Design review of the part built by this model. Coordinates are the model's own, in mm. Face numbers are marked on the shaded views. Give positions to 0.01 mm unless a question says otherwise; leave off trailing zeros. Write each loop counter-clockwise with the first axis right and the second up, starting at its lowest first coordinate (ties: lowest second). Pieces come first, ordered by that corner, then holes.
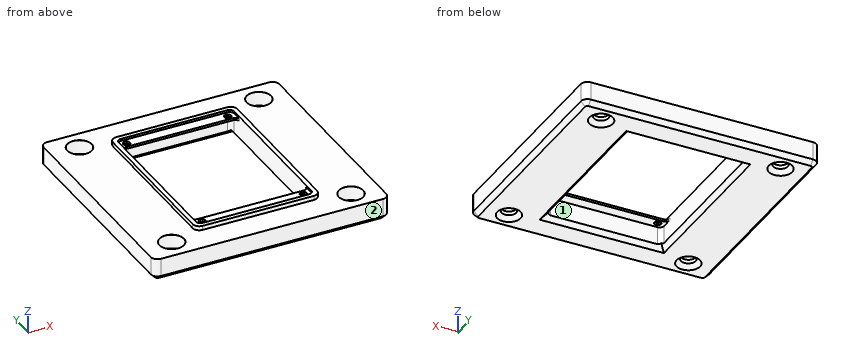
```python
from build123d import *

# Parameters (mm, degrees)
BOSS_EXTRUDE3_DEPTH                          = 10
BOSS_EXTRUDE3_DEPTH_BACK                     = 0.1
SKETCH1_W                                    = 100
SKETCH1_H                                    = 106
SKETCH1_W_2                                  = 76
SKETCH1_H_2                                  = 56
CBORE_FOR_M6_HEX_SOCKET_HEAD_CAP_SCR_2_COUNT = 2
CBORE_FOR_M6_HEX_SOCKET_HEAD_CAP_SCR_2_PITCH = 81
CBORE_FOR_M6_HEX_SOCKET_HEAD_CAP_SCR_3_COUNT = 2
CBORE_FOR_M6_HEX_SOCKET_HEAD_CAP_SCR_3_PITCH = 114.385386776
CBORE_FOR_M6_HEX_SOCKET_HEAD_CAP_SCR_4_COUNT = 2
CBORE_FOR_M6_HEX_SOCKET_HEAD_CAP_SCR_4_PITCH = 80.765194904
SKETCH7_W                                    = 56
SKETCH7_H                                    = 76
BOSS_EXTRUDE4_DEPTH                          = 12
SKETCH8_W                                    = 52
SKETCH8_H                                    = 72
BOSS_EXTRUDE5_DEPTH                          = 1
SKETCH9_W                                    = 52
SKETCH9_H                                    = 72
CUT_EXTRUDE1_DEPTH                           = 1
SKETCH10_W                                   = 52
SKETCH10_H                                   = 62.005454301
CUT_EXTRUDE2_DEPTH                           = 11
SKETCH11_W                                   = 52
SKETCH11_H                                   = 4.999168043
SKETCH11_H_2                                 = 4.995377656
CUT_EXTRUDE3_DEPTH                           = 10
SKETCH12_R                                   = 1.5
CUT_EXTRUDE4_DEPTH                           = 2
SKETCH12_3_R                                 = 1.5
CUT_EXTRUDE5_DEPTH                           = 2
SKETCH14_R                                   = 1.5
CUT_EXTRUDE6_DEPTH                           = 2
SKETCH15_R                                   = 1.5
CUT_EXTRUDE7_DEPTH                           = 2
FILLET2_R                                    = 3
CHAMFER1_SIZE                                = 2
FILLET3_R                                    = 2
FILLET4_R                                    = 2


with BuildPart() as part:
    # Sketch1 → Boss-Extrude3 (new, two sides: drawn at the far end of the back side and taken through both)
    # profile 1 of 4: a face of its own
    with BuildSketch(Plane(origin=(0, 0, 0), x_dir=(0, 1, 0), z_dir=(0, 0, 1)).offset(-BOSS_EXTRUDE3_DEPTH_BACK)):
        with Locations((-4.589836902, -8.848323211)):
            Rectangle(SKETCH1_W, SKETCH1_H)
        with Locations((-4.589836902, -8.848323211)):
            Rectangle(SKETCH1_W_2, SKETCH1_H_2, mode=Mode.SUBTRACT)
    # profile 2 of 4: a face of its own
    with BuildSketch(Plane(origin=(0, 0, 0), x_dir=(0, 1, 0), z_dir=(0, 0, 1)).offset(-BOSS_EXTRUDE3_DEPTH_BACK)):
        Polygon((39.410163098, 31.651676789), (39.410163098, -49.348323211), (45.410163098, -61.848323211), (45.410163098, 44.151676789), align=None)
    # profile 3 of 4: a face of its own
    with BuildSketch(Plane(origin=(0, 0, 0), x_dir=(0, 1, 0), z_dir=(0, 0, 1)).offset(-BOSS_EXTRUDE3_DEPTH_BACK)):
        Polygon((33.410163098, 19.151676789), (33.410163098, -36.848323211), (39.410163098, -49.348323211), (39.410163098, 31.651676789), align=None)
    # profile 4 of 4: a face of its own
    with BuildSketch(Plane(origin=(0, 0, 0), x_dir=(0, 1, 0), z_dir=(0, 0, 1)).offset(-BOSS_EXTRUDE3_DEPTH_BACK)):
        Polygon((45.410163098, -61.848323211), (39.410163098, -49.348323211), (39.410163098, -61.848323211), align=None)
    extrude(amount=BOSS_EXTRUDE3_DEPTH + BOSS_EXTRUDE3_DEPTH_BACK)

    # Sketch6 → CBORE for M6 Hex Socket Head Cap Screw2 (revolve, cut)
    with BuildSketch(Plane(origin=(49.348323211, -45.089836902, 10), x_dir=(0, -1, 0), z_dir=(1, 0, 0))):
        Polygon((0, 0), (0, 10.1), (3.3, 10.1), (3.3, 6.4), (5.5, 6.4), (5.5, 0.025), (5.525, 0), align=None)
    cbore_for_m6_hex_socket_head_cap_screw2 = revolve(axis=Axis((49.348323211, -45.089836902, 16.35), (0, 0, -1)), mode=Mode.SUBTRACT)

    # CBORE for M6 Hex Socket Head Cap Scr 2: CBORE for M6 Hex Socket Head Cap Screw2 ×2
    with Locations(*[(0, i * CBORE_FOR_M6_HEX_SOCKET_HEAD_CAP_SCR_2_PITCH, 0) for i in range(1, CBORE_FOR_M6_HEX_SOCKET_HEAD_CAP_SCR_2_COUNT)]):
        add(cbore_for_m6_hex_socket_head_cap_screw2, mode=Mode.SUBTRACT)

    # CBORE for M6 Hex Socket Head Cap Scr 3: CBORE for M6 Hex Socket Head Cap Screw2 ×2
    with Locations(*[Vector(-0.7060796591298035, 0.7081324134391396, 0) * (i * CBORE_FOR_M6_HEX_SOCKET_HEAD_CAP_SCR_3_PITCH) for i in range(1, CBORE_FOR_M6_HEX_SOCKET_HEAD_CAP_SCR_3_COUNT)]):
        add(cbore_for_m6_hex_socket_head_cap_screw2, mode=Mode.SUBTRACT)

    # CBORE for M6 Hex Socket Head Cap Scr 4: CBORE for M6 Hex Socket Head Cap Screw2 ×2
    with Locations(*[(-i * CBORE_FOR_M6_HEX_SOCKET_HEAD_CAP_SCR_4_PITCH, 0, 0) for i in range(1, CBORE_FOR_M6_HEX_SOCKET_HEAD_CAP_SCR_4_COUNT)]):
        add(cbore_for_m6_hex_socket_head_cap_screw2, mode=Mode.SUBTRACT)

    # Sketch7 → Boss-Extrude4 (add)
    with BuildSketch(Plane(origin=(0, 0, -0.1), x_dir=(1, 0, 0), z_dir=(0, 0, -1))):
        with Locations((8.848323211, 4.589836902)):
            Rectangle(SKETCH7_W, SKETCH7_H)
    extrude(amount=-BOSS_EXTRUDE4_DEPTH)

    # Sketch8 → Boss-Extrude5 (add)
    with BuildSketch(Plane.XY.offset(11.9)):
        with Locations((8.848323211, -4.589836902)):
            Rectangle(SKETCH8_W, SKETCH8_H)
    extrude(amount=-BOSS_EXTRUDE5_DEPTH)

    # Sketch9 → Cut-Extrude1 (cut)
    with BuildSketch(Plane.XY.offset(11.9)):
        with Locations((8.848323211, -4.589836902)):
            Rectangle(SKETCH9_W, SKETCH9_H)
    extrude(amount=-CUT_EXTRUDE1_DEPTH, mode=Mode.SUBTRACT)

    # Sketch10 → Cut-Extrude2 (cut)
    with BuildSketch(Plane.XY.offset(10.9)):
        with Locations((8.848323211, -4.587941709)):
            Rectangle(SKETCH10_W, SKETCH10_H)
    extrude(amount=-CUT_EXTRUDE2_DEPTH, mode=Mode.SUBTRACT)

    # Sketch11 → Cut-Extrude3 (cut)
    with BuildSketch(Plane(origin=(0, 0, -0.1), x_dir=(1, 0, 0), z_dir=(0, 0, -1))):
        with Locations((8.848323211, 38.090252881)):
            Rectangle(SKETCH11_W, SKETCH11_H)
        with Locations((8.848323211, -28.91247427)):
            Rectangle(SKETCH11_W, SKETCH11_H_2)
    extrude(amount=-CUT_EXTRUDE3_DEPTH, mode=Mode.SUBTRACT)

    # Sketch12 → Cut-Extrude4 (cut)
    with BuildSketch(Plane.XY.offset(10.9)):
        with Locations((-13.901676789, 28.660163098)):
            Circle(SKETCH12_R)
    extrude(amount=-CUT_EXTRUDE4_DEPTH, mode=Mode.SUBTRACT)

    # Sketch12_3 → Cut-Extrude5 (cut)
    with BuildSketch(Plane.XY.offset(10.9)):
        with Locations((31.598323211, 28.660163098)):
            Circle(SKETCH12_3_R)
    extrude(amount=-CUT_EXTRUDE5_DEPTH, mode=Mode.SUBTRACT)

    # Sketch14 → Cut-Extrude6 (cut)
    with BuildSketch(Plane.XY.offset(10.9)):
        with Locations((-13.901676789, -37.839836902)):
            Circle(SKETCH14_R)
    extrude(amount=-CUT_EXTRUDE6_DEPTH, mode=Mode.SUBTRACT)

    # Sketch15 → Cut-Extrude7 (cut)
    with BuildSketch(Plane.XY.offset(10.9)):
        with Locations((31.598323211, -37.839836902)):
            Circle(SKETCH15_R)
    extrude(amount=-CUT_EXTRUDE7_DEPTH, mode=Mode.SUBTRACT)

    # Fillet2
    fillet2_edges = [part.edges().sort_by_distance(p)[0] for p in [
        (61.848323211, -54.589836902, 4.95),
        (-44.151676789, -54.589836902, 4.95),
        (-44.151676789, 45.410163098, 4.95),
        (61.848323211, 45.410163098, 4.95),
        (-19.151676789, 33.410163098, 10.95),
        (-19.151676789, -42.589836902, 10.95),
        (36.848323211, -42.589836902, 10.95),
        (36.848323211, 33.410163098, 10.95),
    ]]
    fillet(fillet2_edges, radius=FILLET2_R)

    # Chamfer1
    chamfer1_edges = [part.edges().sort_by_distance(p)[0] for p in [
        (-17.151676789, -4.589836902, -0.1),
        (34.848323211, -4.589836902, -0.1),
        (8.848323211, -40.589836902, -0.1),
        (8.848323211, 31.410163098, -0.1),
        (8.848323211, 45.410163098, -0.1),
        (-44.151676789, -4.589836902, -0.1),
        (61.848323211, -4.589836902, -0.1),
        (8.848323211, -54.589836902, -0.1),
        (-43.272997132, -53.711157246, -0.1),
        (60.969643555, -53.711157246, -0.1),
        (60.969643555, 44.531483441, -0.1),
        (-43.272997132, 44.531483441, -0.1),
        (49.348323211, -41.789836902, -0.1),
        (-31.416871693, -41.789836902, -0.1),
        (-31.416871693, 39.210163098, -0.1),
        (49.348323211, 39.210163098, -0.1),
    ]]
    chamfer(chamfer1_edges, length=CHAMFER1_SIZE)

    # Fillet3
    fillet3_edges = [part.edges().sort_by_distance(p)[0] for p in [
        (34.848323211, -35.590668859, 10.4),
    ]]
    fillet(fillet3_edges, radius=FILLET3_R)

    # Fillet4
    fillet4_edges = [part.edges().sort_by_distance(p)[0] for p in [
        (-17.151676789, -40.589836902, 11.4),
        (-17.151676789, 31.410163098, 11.4),
        (34.848323211, 31.410163098, 11.4),
        (34.848323211, -40.589836902, 11.4),
        (-17.151676789, 26.414785442, 10.4),
        (34.848323211, 26.414785442, 10.4),
        (-17.151676789, -35.590668859, 10.4),
        (-17.151676789, -40.589836902, 5.9),
        (34.848323211, -40.589836902, 5.9),
        (34.848323211, 31.410163098, 5.9),
        (-17.151676789, 31.410163098, 5.9),
    ]]
    fillet(fillet4_edges, radius=FILLET4_R)


solid = part.part
```
(1) Clearance check with flat-ended pins moving along their axes: P1, Ø12, axis at x = 47.5, y = -47.5, coming from the +Z side; P2, Ø5, axis at x = 31.6, y = -37.84, coming from the -Z side; P3, Ø1, axis at y = 2.5, z = 11.5, coming from the -X side. State where each tip first meets the part, or that it passes through.
Resolved:
P1: stops at z = 10
P2: stops at z = 9.9
P3: stops at x = -19.15
(2) Mouldability with a two-part tool opening along X and no side actions: class the marked faces 1 and 2 as pulls with the +X half, pulls with the -X half, needs draft (parallel to the pull), parting line crosses it, or undercut.
Resolved:
face 1: undercut
face 2: needs draft
(3) Consider section A-A, the plane y = 19. Give the boundary of the cut face in (x, z).
Resolved:
outline: (-44.15, 1.9) - (-42.15, -0.1) - (-19.15, -0.1) - (-17.15, 1.9) - (-17.15, 11.9) - (-19.15, 11.9) - (-19.15, 10) - (-44.15, 10) - close; (34.85, 1.9) - (36.85, -0.1) - (59.85, -0.1) - (61.85, 1.9) - (61.85, 10) - (36.85, 10) - (36.85, 11.9) - (34.85, 11.9) - close
(4) Consider section C-C, the plane x = 31.5. Give the number of separate pieces and of enclosed holes in the cut face, then the cut area to 3 significant figures.
Resolved:
separate pieces: 4
enclosed holes: 0
area: 286 mm2
(5) Consider section D-D, the plane z = 5.75. Give the boundary of the cut face in (x, y).
Resolved:
outline: (-44.15, -51.59) arc R3 ccw to (-41.15, -54.59) - (58.85, -54.59) arc R3 ccw to (61.85, -51.59) - (61.85, 42.41) arc R3 ccw to (58.85, 45.41) - (-41.15, 45.41) arc R3 ccw to (-44.15, 42.41) - close; hole circle Ø11 at (-31.42, -45.09); hole circle Ø11 at (-31.42, 35.91); hole (-17.15, -38.59) arc R2 ccw to (-15.15, -40.59) - (32.85, -40.59) arc R2 ccw to (34.85, -38.59) - (34.85, 29.41) arc R2 ccw to (32.85, 31.41) - (-15.15, 31.41) arc R2 ccw to (-17.15, 29.41) - close; hole circle Ø11 at (49.35, -45.09); hole circle Ø11 at (49.35, 35.91)
(6) To check wall thickness, follow L1, parallel to X at y = 22, z = 6.5; L2, parallel to Y at x = -10, z = 5.75; L3, parallel to Y at x = -33.5, z = 5.5. State the ranges of each line that lie inside material, in increasing order.
Resolved:
L1: x = -44.15 to -17.15, 34.85 to 61.85
L2: y = -54.59 to -40.59, 31.41 to 45.41
L3: y = -54.59 to -50.18, -40 to 30.82, 41 to 45.41
(7) Consider section B-B, the plane x = 11.5. Give the boundary of the cut face in (y, z).
Resolved:
outline: (-54.59, 1.9) - (-52.59, -0.1) - (-42.59, -0.1) - (-40.59, 1.9) - (-40.59, 9.9) - (-35.59, 9.9) - (-35.59, 10.9) - (-40.59, 10.9) - (-40.59, 11.9) - (-42.59, 11.9) - (-42.59, 10) - (-54.59, 10) - close; (26.41, 9.9) - (31.41, 9.9) - (31.41, 1.9) - (33.41, -0.1) - (43.41, -0.1) - (45.41, 1.9) - (45.41, 10) - (33.41, 10) - (33.41, 11.9) - (31.41, 11.9) - (31.41, 10.9) - (26.41, 10.9) - close
